```python
from build123d import *

# Parameters (mm, degrees)
SKETCH1_W           = 18
SKETCH1_H           = 129
SKETCH1_W_2         = 8
SKETCH1_H_2         = 2.5
BOSS_EXTRUDE1_DEPTH = 2.5
FILLET1_R           = 1


with BuildPart() as part:
    # Sketch1 → Boss-Extrude1 (new body)
    with BuildSketch(Plane(origin=(0, 0, 0), x_dir=(1, 0, 0), z_dir=(0, 1, 0))):
        Rectangle(SKETCH1_W, SKETCH1_H)
        with Locations((0, 61.25)):
            Rectangle(SKETCH1_W_2, SKETCH1_H_2, mode=Mode.SUBTRACT)
        with Locations((0, -61.25)):
            Rectangle(SKETCH1_W_2, SKETCH1_H_2, mode=Mode.SUBTRACT)
    extrude(amount=BOSS_EXTRUDE1_DEPTH)

    # Fillet1
    fillet1_edges = [part.edges().sort_by_distance(p)[0] for p in [
        (9, 1.25, 64.5),
        (-9, 1.25, 64.5),
        (-9, 1.25, -64.5),
        (9, 1.25, -64.5),
    ]]
    fillet(fillet1_edges, radius=FILLET1_R)


solid = part.part
```
Check sheet for the modelled part. Datum: model origin and axes. Units: mm. A direction names the side the tool comes from. Coordinates: 2 decimals unless noted, no trailing zeros. Write each loop counter-clockwise with the first axis right and the second up, starting at its lowest first coordinate (ties: lowest second). Pieces come first, ordered by that corner, then holes. Notation, with made-up numbers: (76.25, 27.25) -> (100.25, 27.25) arc R25 ccw to (100.25, 45.25) -> close; hole circle Ø7 at (-21, -24.75). An arc over 180 degrees is marked (long way). Use a Markdown table: item, result.
1. Scan line: line 1 along Z through (x, y) = (0, 1.7). Record every from-to range of solid material in increasing order.
Reported:
| item | result |
|---|---|
| line 1 | z = -64.5 to -62.5, -60 to 60, 62.5 to 64.5 |
2. Release check for a two-part mould opening along X. For faces 1 (the flat face through (9, 1, 1)), 2 (the flat face through (-9, 1, 1)), 3 (the flat face through (4, 1, 61)), 4 (the flat face through (0, 1, -64.5)) record: pulls with the +X half, pulls with the -X half, needs draft (parallel to the pull), parting line crosses it, or undercut.
Reported:
| item | result |
|---|---|
| face 1 | pulls with the +X half |
| face 2 | pulls with the -X half |
| face 3 | undercut |
| face 4 | needs draft |
3. Tool access check on faces 5 (the flat face through (0, 1, 64.5)), 6 (the flat face through (0, 1, 62.5)). Record the directions out of +Z, -Z, +X, -X, +Y, -Y that give a thin tool (end or side, any length) a straight path to the whole face; none if there is none.
Reported:
| item | result |
|---|---|
| face 5 | +Z, +X, -X, +Y, -Y |
| face 6 | +Y, -Y |
4. Sectioned sample at A-A (y = 2.05). Enter the section's corners in (x, z).
Reported:
| item | result |
|---|---|
| outline | (-9, -63.5) arc R1 ccw to (-8, -64.5) -> (8, -64.5) arc R1 ccw to (9, -63.5) -> (9, 63.5) arc R1 ccw to (8, 64.5) -> (-8, 64.5) arc R1 ccw to (-9, 63.5) -> close; hole (-4, -62.5) -> (4, -62.5) -> (4, -60) -> (-4, -60) -> close; hole (-4, 60) -> (4, 60) -> (4, 62.5) -> (-4, 62.5) -> close |
